Can you work these out from the model? Positions are in its coordinate system, mm. Coordinates: 2 decimals unless noted, no trailing zeros. Loops run counter-clockwise (first coordinate to the right, second up) from the corner with the lowest first, then second, coordinate; pieces in that order, holes last. Notation, with made-up numbers: (23.25, 66.25) - (27.25, 66.25) arc R18 cw to (27.25, 95.25) - close; hole circle Ø2 at (34, 3.5). An arc over 180 degrees is marked (long way). Put each result on its own line as item: value. Start each with the question number.
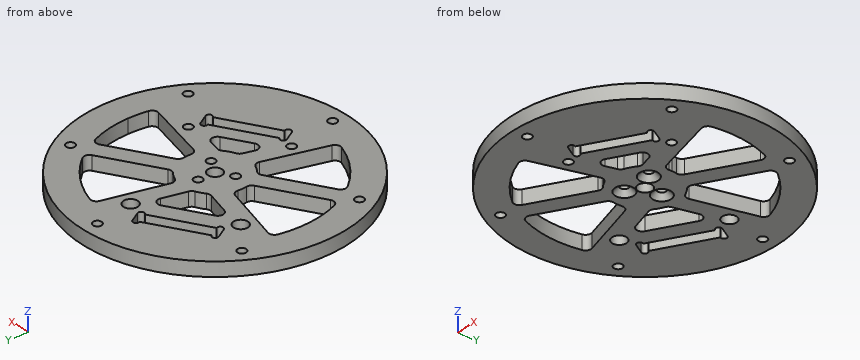
from build123d import *

# Parameters (mm, degrees)
SKETCH_1_R                   = 47
EXTRUDE_1_DEPTH              = 5
SKETCH_2_R                   = 1.525
CUT_EXTRUDE_1_DEPTH          = 25
CUT_EXTRUDE_3_DEPTH          = 10
SKETCH_5_R                   = 1.05
CUT_EXTRUDE_4_DEPTH          = 40
CUT_EXTRUDE_7_DEPTH          = 10
SKETCH_8_R                   = 1.05
CUT_EXTRUDE_8_DEPTH          = 10
SKETCH_11_R                  = 1.525
CUT_EXTRUDE_9_DEPTH          = 10
SKETCH_12_R                  = 1.525
SKETCH_12_R_2                = 2.525
CUT_EXTRUDE_10_DEPTH         = 6.5
SKETCH_13_R                  = 2.5
CUT_EXTRUDE_11_DEPTH         = 50
CUT_EXTRUDE_13_DEPTH         = 50
HOLE_WIZARD_M3_1_D           = 3
HOLE_WIZARD_M3_1_CSINK_D     = 6.6
HOLE_WIZARD_M3_1_CSINK_ANGLE = 90
CUT_EXTRUDE_START            = -50
CUT_EXTRUDE_14_DEPTH         = 50
CUT_EXTRUDE_15_DEPTH         = 50
FILLET_1_R                   = 2


with BuildPart() as part:
    # 草图1 → 凸台-拉伸1 (new body)
    with BuildSketch(Plane.XY):
        Circle(SKETCH_1_R)
    extrude(amount=EXTRUDE_1_DEPTH)

    # 草图2 → 切除-拉伸1 (cut)
    with BuildSketch(Plane.XY.offset(5)):
        with Locations((0, 42)):
            Circle(SKETCH_2_R)
        with Locations((36.373066959, 21)):
            Circle(SKETCH_2_R)
        with Locations((36.373066959, -21)):
            Circle(SKETCH_2_R)
        with Locations((0, -42)):
            Circle(SKETCH_2_R)
        with Locations((-36.373066959, -21)):
            Circle(SKETCH_2_R)
        with Locations((-36.373066959, 21)):
            Circle(SKETCH_2_R)
    extrude(amount=-CUT_EXTRUDE_1_DEPTH, mode=Mode.SUBTRACT)

    # 草图4 → 切除-拉伸3 (cut)
    with BuildSketch(Plane.XY.offset(5)):
        Polygon((22.343618817, -13.600283017), (0.606381183, -26.150283017), (2.656381183, -29.700987172), (24.393618817, -17.150987172), align=None)
    extrude(amount=-CUT_EXTRUDE_3_DEPTH, mode=Mode.SUBTRACT)

    # 草图5 → 切除-拉伸4 (cut)
    with BuildSketch(Plane.XY.offset(5)):
        with Locations((21.434292144, -14.125283017)):
            Circle(SKETCH_5_R)
        with Locations((23.484292144, -17.675987172)):
            Circle(SKETCH_5_R)
        with Locations((1.515707856, -25.625283017)):
            Circle(SKETCH_5_R)
        with Locations((3.565707856, -29.175987172)):
            Circle(SKETCH_5_R)
    extrude(amount=-CUT_EXTRUDE_4_DEPTH, mode=Mode.SUBTRACT)

    # 草图7 → 切除-拉伸7 (cut)
    with BuildSketch(Plane.XY.offset(5)):
        Polygon((-4.906381183, 33.598101489), (-26.643618817, 21.048101489), (-24.593618817, 17.497397334), (-2.856381183, 30.047397334), align=None)
    extrude(amount=-CUT_EXTRUDE_7_DEPTH, mode=Mode.SUBTRACT)

    # 草图8 → 切除-拉伸8 (cut)
    with BuildSketch(Plane.XY.offset(5)):
        with Locations((-23.684292144, 18.022397334)):
            Circle(SKETCH_8_R)
        with Locations((-25.734292144, 21.573101489)):
            Circle(SKETCH_8_R)
        with Locations((-5.815707856, 33.073101489)):
            Circle(SKETCH_8_R)
        with Locations((-3.765707856, 29.522397334)):
            Circle(SKETCH_8_R)
    extrude(amount=-CUT_EXTRUDE_8_DEPTH, mode=Mode.SUBTRACT)

    # 草图11 → 切除-拉伸9 (cut)
    with BuildSketch(Plane.XY.offset(5)):
        with Locations((0, 6)):
            Circle(SKETCH_11_R)
        with Locations((5.196152423, -3)):
            Circle(SKETCH_11_R)
        with Locations((-5.196152423, -3)):
            Circle(SKETCH_11_R)
    extrude(amount=-CUT_EXTRUDE_9_DEPTH, mode=Mode.SUBTRACT)

    # 草图12 → 切除-拉伸10 (cut)
    with BuildSketch(Plane(origin=(0, 0, 0), x_dir=(-1, 0, 0), z_dir=(0, 0, -1))):
        with Locations((2.990381057, -24.820508076)):
            Circle(SKETCH_12_R)
        with Locations((-22.990381057, -9.820508076)):
            Circle(SKETCH_12_R)
        with Locations((-2.106406461, 28.351596989)):
            Circle(SKETCH_12_R_2)
        with Locations((25.606406461, 12.351596989)):
            Circle(SKETCH_12_R_2)
    extrude(amount=-CUT_EXTRUDE_10_DEPTH, mode=Mode.SUBTRACT)

    # 草图13 → 切除-拉伸11 (cut)
    with BuildSketch(Plane(origin=(0, 0, 0), x_dir=(-1, 0, 0), z_dir=(0, 0, -1))):
        Circle(SKETCH_13_R)
    extrude(amount=-CUT_EXTRUDE_11_DEPTH, mode=Mode.SUBTRACT)

    # 草图16 → 切除-拉伸13 (cut)
    with BuildSketch(Plane.XY.offset(5)):
        with BuildLine():
            Line((33.437438845, 15.841012703), (11.114442262, 2.952824616))
            ThreePointArc((11.114442262, 2.952824616), (11.40320319, 1.488944927), (11.5, 0))
            ThreePointArc((11.5, 0), (11.415217398, -1.393847822), (11.162119696, -2.767143635))
            Line((11.162119696, -2.767143635), (35.912906847, -8.90298387))
            ThreePointArc((35.912906847, -8.90298387), (36.727221195, -4.484553861), (37, 0))
            ThreePointArc((37, 0), (36.098374183, 8.11833612), (33.437438845, 15.841012703))
        make_face()
        with BuildLine():
            Line((9.18804638, 35.841035193), (2.855744145, 11.139781209))
            ThreePointArc((2.855744145, 11.139781209), (5.685285819, 9.996375601), (8.114442262, 8.148977039))
            Line((8.114442262, 8.148977039), (30.437438845, 21.037165126))
            ThreePointArc((30.437438845, 21.037165126), (21.150257967, 30.358962234), (9.18804638, 35.841035193))
        make_face()
        with BuildLine():
            ThreePointArc((-11.114442262, -2.952824616), (-11.499758126, 0.074585853), (-11.075205592, 3.096743628))
            Line((-11.075205592, 3.096743628), (-35.633270165, 9.96343602))
            ThreePointArc((-35.633270165, 9.96343602), (-36.866761511, -3.137179579), (-33.437438845, -15.841012703))
            Line((-33.437438845, -15.841012703), (-11.114442262, -2.952824616))
        make_face()
        with BuildLine():
            Line((-10.246243223, -35.552981588), (-3.184643164, -11.050251034))
            ThreePointArc((-3.184643164, -11.050251034), (-5.832810691, -9.911020101), (-8.114442262, -8.148977039))
            Line((-8.114442262, -8.148977039), (-30.437438845, -21.037165126))
            ThreePointArc((-30.437438845, -21.037165126), (-21.597863981, -30.042174879), (-10.246243223, -35.552981588))
        make_face()
    extrude(amount=-CUT_EXTRUDE_13_DEPTH, mode=Mode.SUBTRACT)

    # M3 十字槽沉头木螺钉的锥形沉头孔1 (through all)
    with Locations(Plane(origin=(0, 0, 0), x_dir=(-1, 0, 0), z_dir=(0, 0, -1))):
        with Locations((5.196152423, -3), (-5.196152423, -3), (0, 6)):
            CounterSinkHole(HOLE_WIZARD_M3_1_D / 2, HOLE_WIZARD_M3_1_CSINK_D / 2, counter_sink_angle=HOLE_WIZARD_M3_1_CSINK_ANGLE)

    # 草图19 → 切除-拉伸14 (cut)
    with BuildSketch(Plane(origin=(0, 0, 0), x_dir=(-1, 0, 0), z_dir=(0, 0, -1)).offset(CUT_EXTRUDE_START)):
        with BuildLine():
            Line((21.632488727, 12.278803359), (-0.182488727, 24.873686464))
            Line((-0.182488727, 24.873686464), (3.37580992, 10.993357421))
            ThreePointArc((3.37580992, 10.993357421), (5.75, 9.959292144), (7.832621839, 8.420215859))
            Line((7.832621839, 8.420215859), (21.632488727, 12.278803359))
        make_face()
    extrude(amount=CUT_EXTRUDE_14_DEPTH, mode=Mode.SUBTRACT)

    # 草图20 → 切除-拉伸15 (cut)
    with BuildSketch(Plane(origin=(0, 0, 0), x_dir=(-1, 0, 0), z_dir=(0, 0, -1)).offset(CUT_EXTRUDE_START)):
        with BuildLine():
            Line((-0.324840576, -20.53932787), (-3.0485131, -11.088578262))
            ThreePointArc((-3.0485131, -11.088578262), (-5.75, -9.959292144), (-8.078733917, -8.18437892))
            Line((-8.078733917, -8.18437892), (-17.625159424, -10.550984126))
            Line((-17.625159424, -10.550984126), (-0.324840576, -20.53932787))
        make_face()
    extrude(amount=CUT_EXTRUDE_15_DEPTH, mode=Mode.SUBTRACT)

    # 圆角1
    fillet_1_edges = [part.edges().sort_by_distance(p)[0] for p in [
        (8.114442262, 8.148977039, 2.5),
        (2.855744145, 11.139781209, 2.5),
        (9.18804638, 35.841035193, 2.5),
        (30.437438845, 21.037165126, 2.5),
        (-11.075205592, 3.096743628, 2.5),
        (-11.114442262, -2.952824616, 2.5),
        (-33.437438845, -15.841012703, 2.5),
        (-35.633270165, 9.96343602, 2.5),
        (-8.114442262, -8.148977039, 2.5),
        (-3.184643164, -11.050251034, 2.5),
        (-10.246243223, -35.552981588, 2.5),
        (-30.437438845, -21.037165126, 2.5),
        (11.162119696, -2.767143635, 2.5),
        (11.114442262, 2.952824616, 2.5),
        (33.437438845, 15.841012703, 2.5),
        (35.912906847, -8.90298387, 2.5),
        (-7.832621839, 8.420215859, 2.5),
        (-3.37580992, 10.993357421, 2.5),
        (0.182488727, 24.873686464, 2.5),
        (-21.632488727, 12.278803359, 2.5),
        (8.078733917, -8.18437892, 2.5),
        (3.0485131, -11.088578262, 2.5),
        (0.324840576, -20.53932787, 2.5),
        (17.625159424, -10.550984126, 2.5),
    ]]
    fillet(fillet_1_edges, radius=FILLET_1_R)


solid = part.part
Q1. I want a section at D-D on x = 39. List the corners of the cut face in (y, z) for me, and give its area (3 significant figures).
Q2. I want a section at A-A on y = -21. List the corners of the cut face in (x, z) for me.
Q3. Please list where these lines run through material, in increasing order: line 1 along Y through (x, z) = (-15.5, 4.15); line 2 along Y through (x, z) = (0, 2.1) (3 decimals); line 3 along X through (y, z) = (3, 1.4). Write a range as [from, to].
Q4. I want a section at B-B on y = -42. List the corners of the cut face in (x, z) for me (3 decimals), and give its area (3 significant figures).
Q5. I want a section at C-C on y = 6. List the corners of the cut face in (x, z) for me (3 decimals), and give its area (3 significant figures).
Q6. Will these pins go through, and if not, where does the flat tip stop? pin 1 (5 mm diameter, centred on x = -5.2, y = -3, fed in from -Z); pin 2 (2.5 mm diameter, centred on x = -36.37, y = 21, fed in from -Z).
Calculated:
1. outline: (-26.23, 0) - (26.23, 0) - (26.23, 5) - (-26.23, 5) - close
1. area: 262 mm2
2. outline: (-42.05, 0) - (-37.9, 0) - (-37.9, 5) - (-42.05, 5) - close; (-34.85, 0) - (-29.39, 0) - (-29.39, 5) - (-34.85, 5) - close; (-6.05, 0) - (9.53, 0) - (9.53, 5) - (-6.05, 5) - close; (17.73, 0) - (34.85, 0) - (34.85, 5) - (17.73, 5) - close; (37.9, 0) - (42.05, 0) - (42.05, 5) - (37.9, 5) - close
3. line 1: [-44.37, -33.6], [-12.41, -5.48], [4.33, 10.56], [15.82, 22.75], [27.48, 44.37]
3. line 2: [-47, -43.525], [-40.475, -2.5], [2.5, 4.475], [7.525, 26.959], [29.744, 40.475], [43.525, 47]
3. line 3: [-46.9, -36.88], [-11.9, 11.66], [36.88, 46.9]
4. outline: (-21.095, 0) - (-1.525, 0) - (-1.525, 5) - (-21.095, 5) - close; (1.525, 0) - (21.095, 0) - (21.095, 5) - (1.525, 5) - close
4. area: 196 mm2
5. outline: (-46.615, 0) - (-36.51, 0) - (-36.51, 5) - (-46.615, 5) - close; (-21.458, 0) - (-3.3, 0) - (-1.525, 1.775) - (-1.525, 5) - (-21.458, 5) - close; (1.525, 1.775) - (3.3, 0) - (16.392, 0) - (16.392, 5) - (1.525, 5) - close; (36.51, 0) - (46.615, 0) - (46.615, 5) - (36.51, 5) - close
5. area: 272 mm2
6. pin 1: z = 0.8
6. pin 2: through
